Autodesk Inventor part; units mm, degrees
ref_plane "YZ Plane" through (0, 0, 0) normal (1, 0, 0) x (0, 1, 0)
ref_plane "XZ Plane" through (0, 0, 0) normal (0, 1, 0) x (-1, 0, 0)
ref_plane "XY Plane" through (0, 0, 0) normal (0, 0, 1) x (1, 0, 0)
sketch "Skizze1" plane through (0, 0, 0) normal (0, 0, 1) x (1, 0, 0)
  line L0 (-53, 32.5) -> (53, 32.5)
  line L1 (55, 30.5) -> (55, -30.5)
  line L2 (53, -32.5) -> (-53, -32.5)
  line L3 (-55, -30.5) -> (-55, 30.5)
  line L4 (-55, 32.5) -> (55, -32.5) construction
  line L5 (55, 32.5) -> (-55, -32.5) construction
  arc A0 (-53, 32.5) -> (-55, 30.5) centre (-53, 30.5) ccw
  arc A1 (55, 30.5) -> (53, 32.5) centre (53, 30.5) ccw
  arc A2 (53, -32.5) -> (55, -30.5) centre (53, -30.5) ccw
  arc A3 (-55, -30.5) -> (-53, -32.5) centre (-53, -30.5) ccw
  point P0 (0, 0)
  dimension "d0" = 110
  dimension "d1" = 65
  dimension "d2" = 2
extrude "Extrusion1" add sketch "Skizze1" along normal blind 1.5
sketch "Skizze2" plane through (0, 0, 1.5) normal (0, 0, 1) x (1, 0, 0)
  circle A0 centre (-51, 28.5) radius 2
  circle A1 centre (-51, -28.5) radius 2
  circle A2 centre (51, -28.5) radius 2
  circle A3 centre (51, 28.5) radius 2
  line L0 (-55, 30.5) -> (-55, -30.5)
  line L1 (-53, -32.5) -> (53, -32.5)
  point P0 (0, 0)
  dimension "d5" = 4
  dimension "d6" = 4
  dimension "d7" = 4
  dimension "d8" = 4
  dimension "d9" = 102
  dimension "d10" = 102
  dimension "d11" = 57
  dimension "d12" = 57
  dimension "d13" = 4
  dimension "d14" = 4
  dimension "d15" = 4
  dimension "d16" = 4
extrude "Extrusion2" cut sketch "Skizze2" against normal up to next
sketch "Skizze3" plane through (0, 0, 1.5) normal (0, 0, 1) x (1, 0, 0)
  line L0 (-40, -29) -> (40, -29)
  line L1 (40, -29) -> (40, 29)
  line L2 (40, 29) -> (-40, 29)
  line L3 (-40, 29) -> (-40, -29)
  line L4 (53, 32.5) -> (-53, 32.5)
  line L5 (-55, 30.5) -> (-55, -30.5)
  point P0 (0, 0)
  dimension "d19" = 80
  dimension "d20" = 58
  dimension "d21" = 3.5
  dimension "d22" = 15
extrude "Extrusion3" add sketch "Skizze3" along normal blind 4
sketch "Skizze4" plane through (0, 0, 5.5) normal (0, 0, 1) x (1, 0, 0)
  line L0 (-38, -26) -> (34, -26)
  line L1 (34, -26) -> (34, 27)
  line L2 (34, 27) -> (-38, 27)
  line L3 (-38, 27) -> (-38, -26)
  line L4 (-40, 29) -> (-40, -29)
  line L5 (40, 29) -> (-40, 29)
  point P0 (0, 0)
  dimension "d25" = 72
  dimension "d26" = 53
  dimension "d27" = 2
  dimension "d28" = 2
extrude "Extrusion4" cut sketch "Skizze4" against normal blind 0.3
sketch "Skizze5" plane through (0, 0, 0) normal (0, 0, -1) x (-1, 0, 0)
  line L0 (55, -30.5) -> (55, 30.5)
  line L1 (55, -26.5) -> (41.5, -26.5)
  line L2 (41.5, -26.5) -> (41.5, -12)
  line L3 (41.5, -12) -> (55, -12)
  line L4 (55, -12) -> (55, -26.5)
  line L5 (-53, -32.5) -> (53, -32.5)
  point P0 (0, 0)
  dimension "d31" = 14.5
  dimension "d32" = 6
  dimension "d33" = 13.5
extrude "Extrusion5" add sketch "Skizze5" along normal blind 8
sketch "Skizze6" plane through (0, 0, 0) normal (0, 0, -1) x (-1, 0, 0)
  line L0 (55, 30.5) -> (55, -30.5)
  line L1 (55, 24.5) -> (25, 24.5)
  line L2 (25, 24.5) -> (25, -5.5)
  line L3 (25, -5.5) -> (55, -5.5)
  line L4 (55, -5.5) -> (55, 24.5)
  line L5 (53, 32.5) -> (-53, 32.5)
  point P0 (0, 0)
  dimension "d36" = 30
  dimension "d37" = 30
  dimension "d38" = 8
extrude "Extrusion6" add sketch "Skizze6" along normal blind 2.8
properties part number "MKF TFT32" material "Edelstahl, 440C"
Geometry check sheet. Reference: the model listing, model coordinates, mm. A direction names the side the tool comes from. Give positions to 0.01 mm unless a question says otherwise; leave off trailing zeros. Order: outer loops, then holes, each group sorted by start corner. A loop starts at its lowest first (then second) coordinate and runs counter-clockwise, first axis right, second up.
1. Thickness scan on L1, parallel to Y at x = 51, z = 1; L2, parallel to Y at x = -28.5, z = 5.25; L3, parallel to Y at x = -18, z = 2.5. Record the ranges inside material, lowest first.
2. Section check C-C, the plane x = 29.5. Enter the section's corners in (y, z).
3. Access from +Z, -Z, +X, -X, +Y, -Y to the whole of each face (thin tool, end or side, straight path). Record for faces 4 (the face through (-40, 24.5, -1)), 5 (the face through (-25, 10, -1)), 6 (the face through (-48, -12, -4)).
4. Release check for a two-part mould opening along X. For faces 1 (the face through (0, 31, 1.5)), 2 (the face through (-41.5, -19, -4)), 3 (the face through (-51.434, 26.548, 0.76)) record: pulls with the +X half, pulls with the -X half, needs draft (parallel to the pull), parting line crosses it, or undercut.
5. Section check A-A, the plane z = -1.75. Enter the section's corners in (x, y).
6. Gauge pin test, flat ends, axial feed: pin 1 Ø3 at (x, y) = (-51, -28.5) entering from -Z; pin 2 Ø5 at (x, y) = (22.5, 4.5) entering from +Z; pin 3 Ø0.8 at (x, z) = (-47.5, -1) entering from -Y; pin 4 Ø12 at (x, y) = (5, 6.5) entering from -Z. Record the tip position at first contact, or that the pin passes through.
7. Section check D-D, the plane x = 43. Enter the section's corners in (y, z).
8. Section check B-B, the plane y = 7.5. Enter the section's corners in (x, z), and give its area (3 significant figures).
Values follow:
1. L1: y = -32.5 to -30.5, -26.5 to 26.5, 30.5 to 32.5
1. L2: y = -29 to -26, 27 to 29
1. L3: y = -29 to 29
2. outline: (-32.5, 0) - (32.5, 0) - (32.5, 1.5) - (29, 1.5) - (29, 5.5) - (27, 5.5) - (27, 5.2) - (-26, 5.2) - (-26, 5.5) - (-29, 5.5) - (-29, 1.5) - (-32.5, 1.5) - close
3. face 4: -Z, +X, -X, +Y
3. face 5: -Z, +X, +Y, -Y
3. face 6: -Z, +X, -X
4. face 1: needs draft
4. face 2: pulls with the +X half
4. face 3: undercut
5. outline: (-55, -26.5) - (-41.5, -26.5) - (-41.5, -12) - (-55, -12) - close; (-55, -5.5) - (-25, -5.5) - (-25, 24.5) - (-55, 24.5) - close
6. pin 1: passes through
6. pin 2: stops at z = 5.2
6. pin 3: stops at y = -26.5
6. pin 4: stops at z = 0
7. outline: (-32.5, 0) - (32.5, 0) - (32.5, 1.5) - (-32.5, 1.5) - close
8. outline: (-55, -2.8) - (-25, -2.8) - (-25, 0) - (55, 0) - (55, 1.5) - (40, 1.5) - (40, 5.5) - (34, 5.5) - (34, 5.2) - (-38, 5.2) - (-38, 5.5) - (-40, 5.5) - (-40, 1.5) - (-55, 1.5) - close
8. area: 547 mm2
